Design review of the part built by this model. Coordinates are the model's own, in mm. A direction names the side the tool comes from. Round coordinates to 2 decimals unless told otherwise and drop trailing zeros. Order: outer loops, then holes, each group sorted by start corner. A loop starts at its lowest first (then second) coordinate and runs counter-clockwise, first axis right, second up. Notation, with made-up numbers: (81.25, -40) - (128.25, -40) arc R31 cw to (128.25, -6) - close; hole circle Ø1 at (25, 18). An arc over 180 degrees is marked (long way). Write item = value, one per line.
from build123d import *

# Parameters (mm, degrees)
EXTRUDE_2_DEPTH = 160
SHELL_2_T       = -4


with BuildPart() as part:
    # 草图1 → 凸台-拉伸2 (new, symmetric)
    with BuildSketch(Plane(origin=(0, 0, 0), x_dir=(1, 0, 0), z_dir=(0, 1, 0))):
        Polygon((200, 0), (0, 0), (-150, 0), (-150, -150), (175, -150), align=None)
    extrude(amount=EXTRUDE_2_DEPTH, both=True)

    # 抽壳2
    shell_2_openings = [part.faces().sort_by_distance(p)[0] for p in [
        (25, 0, 0),
    ]]
    offset(amount=SHELL_2_T, openings=shell_2_openings, kind=Kind.INTERSECTION)


solid = part.part
Item 1: Take a section at B-B, the plane x = 91.5. State the section outline as (y, z) points, and give its area (3 significant figures).
Data:
outline = (-160, 0) - (-156, 0) - (-156, 146) - (156, 146) - (156, 0) - (160, 0) - (160, 150) - (-160, 150) - close
area = 2,450 mm2
Item 2: The part is to be moulded in two halves that separate along X. For faces 3 (the face through (10, 2, 150)), 4 (the face through (-146, 2, 72)), 5 (the face through (187.325, 2.24, 76.05)), 6 (the face through (11, 2, 146)), say which applies: +X half, -X half, draft (parallel to the pull), parting line (faces both ways), or undercut.
Data:
face_3 = draft
face_4 = undercut
face_5 = +X half
face_6 = undercut
Item 3: Take a section at C-C, the plane y = 25. State the section outline as (x, z) points, and give its area (3 significant figures).
Data:
outline = (-150, 0) - (-146, 0) - (-146, 146) - (171.61, 146) - (195.94, 0) - (200, 0) - (175, 150) - (-150, 150) - close
area = 2,480 mm2
Item 4: Take a section at D-D, the plane z = 99. State the section outline as (x, y) points, and give its area (3 significant figures).
Data:
outline = (-150, -160) - (183.5, -160) - (183.5, 160) - (-150, 160) - close; hole (-146, -156) - (179.44, -156) - (179.44, 156) - (-146, 156) - close
area = 5,180 mm2
Item 5: Insertion check: P1, Ø5, axis at x = 84, y = -92, coming from the -Z side. The pin has a flat end and moves straight along its axis. Give the tip position at first contact, or say it passes through.
Data:
P1 = 146
Item 6: For line 1 along Y through (x, z) = (31.5, 16); line 2 along X through (y, z) = (-59, 72); line 3 along X through (y, z) = (61, 9.5), list the stretches that pass through material, from the lowest coordinate up. Write a range as [from, to].
Data:
line_1 = [-160, -156], [156, 160]
line_2 = [-150, -146], [183.94, 188]
line_3 = [-150, -146], [194.36, 198.42]
Item 7: For faces 1 (the face through (-150, 2, 74)), 2 (the face through (23, 156, 72)), list the 3-axis set-ups (+Z, -Z, +X, -X, +Y, -Y) from which the entire face can be reached by the end or side of a thin tool; tool diameter is ignored.
Data:
face_1 = +Z, -Z, -X, +Y, -Y
face_2 = -Z
Item 8: Take a section at A-A, the plane z = 28. State the section outline as (x, y) points.
Data:
outline = (-150, -160) - (195.33, -160) - (195.33, 160) - (-150, 160) - close; hole (-146, -156) - (191.28, -156) - (191.28, 156) - (-146, 156) - close
